Read the model definition and answer for the solid it produces. Units are mm, in the model's axes. A direction names the side the tool comes from. Round coordinates to 2 decimals unless told otherwise and drop trailing zeros. Order: outer loops, then holes, each group sorted by start corner. A loop starts at its lowest first (then second) coordinate and runs counter-clockwise, first axis right, second up. Notation, with made-up numbers: (51.25, -30) -> (65.25, -30) arc R33 cw to (65.25, 1) -> close; hole circle Ø9 at (46, 74.25). An arc over 180 degrees is marked (long way). Answer as a JSON object with one key per item and string values. Group by question number.
Item 1: Section C-C, the plane y = -31 is taken. Write down the section's boundary in (x, z), plus the area to 3 significant figures.
Item 2: Given P1, Ø11.5, axis at y = -27, z = 27.5, coming from the -X side; P2, Ø14, axis at y = -21.5, z = -23.5, coming from the +X side; P3, Ø4.5, axis at y = -32.5, z = 32, coming from the +X side, each flat-ended and moving along its own axis, determine where each tip first touches the part or whether it passes through.
Item 3: Section B-B, the plane z = -23.5 is taken. Write down the section's boundary in (x, y).
Item 4: Section D-D, the plane z = 33 is taken. Write down the section's boundary in (x, y), plus the area to 3 significant figures.
Item 5: Section A-A, the plane y = -19 is taken. Write down the section's boundary in (x, z), plus the area to 3 significant figures.
Item 6: For faces 4 (the flat face through (55.237, -28.353, -10.651)), 5 (the flat face through (63.063, -28, -26)), 6 (the flat face through (7.6, -28.4, -10.4)), determine the directions among +Z, -Z, +X, -X, +Y, -Y from which every point of the face is accessible in a straight line to the end or side of a thin tool.
Item 7: Consider probe 1 along Z at (x, y) = (28, -35); probe 2 along X at (y, z) = (-21, -21); probe 3 along Y at (x, z) = (26.5, 22). Determine where each line is inside the solid, lowest interval first. Write a range as from..to.
Item 8: The mould has two halves that part along Y. Classify faces 1 (the cylindrical face through (26.633, -24.41, 30.095)), 2 (the flat face through (31, -44.45, 30)), 3 (the flat face through (94.686, -6, -22)): pulls with the +Y half, pulls with the -Y half, needs draft (parallel to the pull), parting line crosses it, or undercut.
from build123d import *

# Parameters (mm, degrees)
F1_DEPTH = 12.7
F2_W     = 31.75
F2_H     = 14.224
F3_DEPTH = 31.75
F4_R     = 6.35
F5_DEPTH = 25.4


with BuildPart() as f1:
    # F0 (on Front) → F1 (new body)
    with BuildSketch(Plane.XZ):
        Polygon((-32.059978, -10.644176), (-32.059978, -32.742176), (94.686022, -32.742176), (94.686022, -10.644176), (47.188022, 37.107824), (15.438022, 37.107824), align=None)
    extrude(amount=F1_DEPTH)

    # F2 (on face) → F3 (join)
    with BuildSketch(Plane.XZ.offset(12.7)):
        with Locations((31.313022, 29.995824)):
            Rectangle(F2_W, F2_H)
        Polygon((-0.436978, -20.042176), (-0.436978, -32.742176), (63.063022, -32.742176), (63.063022, -20.042176), (47.188022, -0.992176), (15.438022, -0.992176), align=None)
    extrude(amount=F3_DEPTH)

    # F4 (on face) → F5 (cut)
    with BuildSketch(Plane.XY.offset(37.107824)):
        with Locations((31.313022, -28.702)):
            Circle(F4_R)
    extrude(amount=-F5_DEPTH, mode=Mode.SUBTRACT)


solid = f1.part
Values found:
{
 "1": {"outline": "(-0.44, -32.74) -> (63.06, -32.74) -> (63.06, -20.04) -> (47.19, -0.99) -> (15.44, -0.99) -> (-0.44, -20.04) -> close; (15.44, 22.88) -> (25.39, 22.88) -> (25.39, 37.11) -> (15.44, 37.11) -> close; (37.23, 22.88) -> (47.19, 22.88) -> (47.19, 37.11) -> (37.23, 37.11) -> close", "area": "2,000 mm2"},
 "2": {"P1": "x = 15.44", "P2": "x = 63.06", "P3": "x = 47.19"},
 "3": {"outline": "(-32.06, -12.7) -> (-0.44, -12.7) -> (-0.44, -44.45) -> (63.06, -44.45) -> (63.06, -12.7) -> (94.69, -12.7) -> (94.69, 0) -> (-32.06, 0) -> close"},
 "4": {"outline": "(11.35, -12.7) -> (15.44, -12.7) -> (15.44, -44.45) -> (47.19, -44.45) -> (47.19, -12.7) -> (51.27, -12.7) -> (51.27, 0) -> (11.35, 0) -> close; hole circle Ø12.7 at (31.31, -28.7)", "area": "1,390 mm2"},
 "5": {"outline": "(-0.44, -32.74) -> (63.06, -32.74) -> (63.06, -20.04) -> (47.19, -0.99) -> (15.44, -0.99) -> (-0.44, -20.04) -> close; (15.44, 22.88) -> (47.19, 22.88) -> (47.19, 37.11) -> (15.44, 37.11) -> close", "area": "2,170 mm2"},
 "6": {"face 4": "+Z, +X, -Y", "face 5": "+Z, -Z, +X, -Y", "face 6": "+Z, -X, -Y"},
 "7": {"probe 1": "-32.74..-0.99, 22.88..37.11", "probe 2": "-0.44..63.06", "probe 3": "-12.7..0"},
 "8": {"face 1": "undercut", "face 2": "pulls with the -Y half", "face 3": "needs draft"}
}
